Verification items for the finished model (mm, model axes). Face numbers are marked on the shaded views. A direction names the side the tool comes from. Coordinates: 2 decimals unless noted, no trailing zeros. Order: outer loops, then holes, each group sorted by start corner. A loop starts at its lowest first (then second) coordinate and runs counter-clockwise, first axis right, second up. Notation, with made-up numbers: (79.5, 61.5) - (116.5, 61.5) arc R5 cw to (116.5, 65.5) - close; hole circle Ø5 at (20, -20.75). An arc over 180 degrees is marked (long way). Answer as CSV lines item,"result". Start each with the question number.
1. Go/stop test with flat-tipped pins: pin 1 (12 mm diameter, centred on x = 20, z = -19, fed in from -Y); pin 2 (6 mm diameter, centred on x = 4, z = -38, fed in from +Y); pin 3 (1 mm diameter, centred on y = -3.5, z = -27, fed in from +X); pin 4 (0.6 mm diameter, centred on x = -10, y = -2.5, fed in from -Z). Record where each tip stops, or that it passes through.
2. Material ranges on L1, parallel to Z at x = -12.5, y = -2.3; L2, parallel to Y at x = -27, z = 0.5; L3, parallel to Z at x = -22.5, y = -3.3, recorded low to high. Write a range as [from, to].
3. Set-up check for the marked faces 1, 2, 3 and 4: record each of +Z, -Z, +X, -X, +Y, -Y from which the full face is reachable in a straight line by a thin tool's end or side.
4. Section check B-B (z = 19). Record the cut outline in (x, y).
5. Section check A-A (x = 10). Record the cut outline in (y, z).
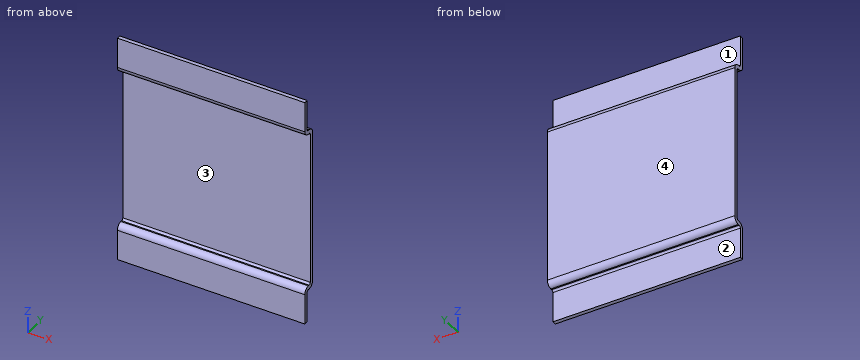
from build123d import *

# Parameters (mm, degrees)
SKETCH1_W                      = 73
SKETCH1_H                      = 64
BASE_FLANGE1_DEPTH             = 1.5
EDGE_FLANGE1_STRIP_W           = 7.4732
EDGE_FLANGE1_STRIP_H           = 1.5
EDGE_FLANGE1_STRIP_CUT_DEPTH   = 73
EDGE_FLANGE1_STRIP_2_W         = 7.4732
EDGE_FLANGE1_STRIP_2_H         = 1.5
EDGE_FLANGE1_STRIP_CUT_2_DEPTH = 73
EDGE_FLANGE1_DEPTH             = 73
EDGE_FLANGE1_BEND_DEPTH        = 73
EDGE_FLANGE2_STRIP_W           = 7.4732
EDGE_FLANGE2_STRIP_H           = 1.5
EDGE_FLANGE2_STRIP_CUT_DEPTH   = 73
EDGE_FLANGE2_STRIP_2_W         = 7.4732
EDGE_FLANGE2_STRIP_2_H         = 1.5
EDGE_FLANGE2_STRIP_CUT_2_DEPTH = 73
EDGE_FLANGE2_DEPTH             = 73
EDGE_FLANGE2_BEND_DEPTH        = 73


# Sheet-metal steps are written as plain solids
with BuildPart() as part:
    # Sketch1 → Base-Flange1 (new body)
    with BuildSketch(Plane(origin=(0, 0, 0), x_dir=(1, 0, 0), z_dir=(0, 1, 0))):
        Rectangle(SKETCH1_W, SKETCH1_H)
    extrude(amount=-BASE_FLANGE1_DEPTH)

    # Edge-Flange1 strip (across the edge) → Edge-Flange1 strip cut (cut)
    with BuildSketch(Plane(origin=(36.5, -1.5, 32), x_dir=(0, 0, -1), z_dir=(-1, 0, 0))):
        with Locations((-1.5, -0.75)):
            Rectangle(EDGE_FLANGE1_STRIP_W, EDGE_FLANGE1_STRIP_H)
    extrude(amount=EDGE_FLANGE1_STRIP_CUT_DEPTH, mode=Mode.SUBTRACT)

    # Edge-Flange1 strip 2 (across the edge) → Edge-Flange1 strip cut 2 (cut)
    with BuildSketch(Plane(origin=(-36.5, -1.5, -32), x_dir=(0, 0, 1), z_dir=(1, 0, 0))):
        with Locations((-1.5, -0.75)):
            Rectangle(EDGE_FLANGE1_STRIP_2_W, EDGE_FLANGE1_STRIP_2_H)
    extrude(amount=EDGE_FLANGE1_STRIP_CUT_2_DEPTH, mode=Mode.SUBTRACT)

    # Edge-Flange1 section (across the edge) → Edge-Flange1 (add)
    with BuildSketch(Plane(origin=(36.5, -1.5, 32), x_dir=(0, 0, -1), z_dir=(-1, 0, 0))):
        with BuildLine():
            Line((0, 0.7366), (0, 3.5))
            Line((0, 3.5), (1.5, 3.5))
            Line((1.5, 3.5), (1.5, 0.7366))
            ThreePointArc((1.5, 0.7366), (1.715745145, 0.215745145), (2.2366, 0))
            Line((2.2366, 0), (2.2366, -1.5))
            ThreePointArc((2.2366, -1.5), (0.655084973, -0.844915027), (0, 0.7366))
        make_face()
    extrude(amount=EDGE_FLANGE1_DEPTH)

    # Edge-Flange1 section 2 (across the edge) → Edge-Flange1 bend (add)
    with BuildSketch(Plane(origin=(-36.5, -1.5, -32), x_dir=(0, 0, 1), z_dir=(1, 0, 0))):
        with BuildLine():
            Line((0, 0.7366), (0, 3.5))
            Line((0, 3.5), (1.5, 3.5))
            Line((1.5, 3.5), (1.5, 0.7366))
            ThreePointArc((1.5, 0.7366), (1.715745145, 0.215745145), (2.2366, 0))
            Line((2.2366, 0), (2.2366, -1.5))
            ThreePointArc((2.2366, -1.5), (0.655084973, -0.844915027), (0, 0.7366))
        make_face()
    extrude(amount=EDGE_FLANGE1_BEND_DEPTH)

    # Edge-Flange2 strip (across the edge) → Edge-Flange2 strip cut (cut)
    with BuildSketch(Plane(origin=(-36.5, -5, 32), x_dir=(0, 1, 0), z_dir=(1, 0, 0))):
        with Locations((-1.5, -0.75)):
            Rectangle(EDGE_FLANGE2_STRIP_W, EDGE_FLANGE2_STRIP_H)
    extrude(amount=EDGE_FLANGE2_STRIP_CUT_DEPTH, mode=Mode.SUBTRACT)

    # Edge-Flange2 strip 2 (across the edge) → Edge-Flange2 strip cut 2 (cut)
    with BuildSketch(Plane(origin=(36.5, -5, -32), x_dir=(0, 1, 0), z_dir=(-1, 0, 0))):
        with Locations((-1.5, -0.75)):
            Rectangle(EDGE_FLANGE2_STRIP_2_W, EDGE_FLANGE2_STRIP_2_H)
    extrude(amount=EDGE_FLANGE2_STRIP_CUT_2_DEPTH, mode=Mode.SUBTRACT)

    # Edge-Flange2 section (across the edge) → Edge-Flange2 (add)
    with BuildSketch(Plane(origin=(-36.5, -5, 32), x_dir=(0, 1, 0), z_dir=(1, 0, 0))):
        with BuildLine():
            Line((0, 0.7366), (0, 12.5))
            Line((0, 12.5), (1.5, 12.5))
            Line((1.5, 12.5), (1.5, 0.7366))
            ThreePointArc((1.5, 0.7366), (1.715745145, 0.215745145), (2.2366, 0))
            Line((2.2366, 0), (2.2366, -1.5))
            ThreePointArc((2.2366, -1.5), (0.655084973, -0.844915027), (0, 0.7366))
        make_face()
    extrude(amount=EDGE_FLANGE2_DEPTH)

    # Edge-Flange2 section 2 (across the edge) → Edge-Flange2 bend (add)
    with BuildSketch(Plane(origin=(36.5, -5, -32), x_dir=(0, 1, 0), z_dir=(-1, 0, 0))):
        with BuildLine():
            Line((0, 0.7366), (0, 12.5))
            Line((0, 12.5), (1.5, 12.5))
            Line((1.5, 12.5), (1.5, 0.7366))
            ThreePointArc((1.5, 0.7366), (1.715745145, 0.215745145), (2.2366, 0))
            Line((2.2366, 0), (2.2366, -1.5))
            ThreePointArc((2.2366, -1.5), (0.655084973, -0.844915027), (0, 0.7366))
        make_face()
    extrude(amount=EDGE_FLANGE2_BEND_DEPTH)


solid = part.part
Evaluation:
1,pin 1,"stops at y = -1.5"
1,pin 2,"stops at y = -3.5"
1,pin 3,"passes through"
1,pin 4,"stops at z = -32"
2,L1,"z = [-32, -30.5], [30.5, 32]"
2,L2,"y = [-1.5, 0]"
2,L3,"z = [-32.23, -30.57], [30.57, 32.23]"
3,face 1,"+Z, +X, -X, +Y"
3,face 2,"-Z, +X, -X, +Y"
3,face 3,"+X, -X, -Y"
3,face 4,"+Z, -Z, +X, -X, +Y"
4,outline,"(-36.5, -1.5) - (36.5, -1.5) - (36.5, 0) - (-36.5, 0) - close"
5,outline,"(-5, -44.5) - (-3.5, -44.5) - (-3.5, -32.74) arc R0.74 cw to (-2.76, -32) - (-2.24, -32) arc R2.24 ccw to (0, -29.76) - (0, 29.76) arc R2.24 ccw to (-2.24, 32) - (-2.76, 32) arc R0.74 cw to (-3.5, 32.74) - (-3.5, 44.5) - (-5, 44.5) - (-5, 32.74) arc R2.24 ccw to (-2.76, 30.5) - (-2.24, 30.5) arc R0.74 cw to (-1.5, 29.76) - (-1.5, -29.76) arc R0.74 cw to (-2.24, -30.5) - (-2.76, -30.5) arc R2.24 ccw to (-5, -32.74) - close"
